```python
from build123d import *

# Parameters (mm, degrees)
BOSS_EXTRUDE1_DEPTH = 65
CUT_EXTRUDE1_DEPTH  = 40
CUT_EXTRUDE4_DEPTH  = 22.5
SKETCH6_R           = 12.5
SKETCH6_R_2         = 5
BOSS_EXTRUDE2_DEPTH = 12
CHAMFER1_SIZE       = 5
FILLET1_R           = 1
SKETCH7_R           = 1
CUT_EXTRUDE5_DEPTH  = 66


with BuildPart() as part:
    # Sketch1 → Boss-Extrude1 (new body, symmetric)
    with BuildSketch(Plane.XY):
        with BuildLine():
            Line((0, 0), (0, -25.554938316))
            ThreePointArc((0, -25.554938316), (-2.359933303, -32.007021768), (-8.325876175, -35.413807897))
            Line((-8.325876175, -35.413807897), (-67.775097409, -45.508814922))
            ThreePointArc((-67.775097409, -45.508814922), (-71.838201048, -44.399413479), (-73.612159322, -40.579380131))
            Line((-73.612159322, -40.579380131), (-73.612159322, -6.5))
            Line((-73.612159322, -6.5), (-29.367881905, -6.5))
            ThreePointArc((-29.367881905, -6.5), (-23.632117541, -4.691520443), (-19.970955697, 0.079798567))
            Line((-19.970955697, 0.079798567), (-20, 0))
            Line((-20, 0), (0, 0))
        make_face()
    extrude(amount=BOSS_EXTRUDE1_DEPTH, both=True)

    # Sketch2 → Cut-Extrude1 (cut, symmetric)
    with BuildSketch(Plane.XY):
        with BuildLine():
            Line((-20, 0), (-19.970955697, 0.079798567))
            ThreePointArc((-19.970955697, 0.079798567), (-20.672372291, -1.438432196), (-21.617003148, -2.818534521))
            Line((-21.617003148, -2.818534521), (-12.102051753, -36.055036129))
            Line((-12.102051753, -36.055036129), (-8.325876175, -35.413807897))
            ThreePointArc((-8.325876175, -35.413807897), (-2.359933303, -32.007021768), (0, -25.554938316))
            Line((0, -25.554938316), (0, 0))
            Line((0, 0), (-20, 0))
        make_face()
    extrude(amount=CUT_EXTRUDE1_DEPTH, both=True, mode=Mode.SUBTRACT)

    # Sketch5 → Cut-Extrude4 (cut, symmetric)
    with BuildSketch(Plane(origin=(0, -6.5, 0), x_dir=(1, 0, 0), z_dir=(0, 1, 0))):
        Polygon((-73.612159322, 40), (-29.401702386, 40), (0, 40), (0, -40), (-29.367881905, -40), (-73.612159322, -40), align=None)
    extrude(amount=CUT_EXTRUDE4_DEPTH, both=True, mode=Mode.SUBTRACT)

    # Sketch6 → Boss-Extrude2 (add)
    with BuildSketch(Plane(origin=(5.611689276, -33.047085202, 0), x_dir=(0.985886958, 0.167412383, 0), z_dir=(0.167412383, -0.985886958, 0))):
        with Locations((-42.967314491, 0)):
            Circle(SKETCH6_R)
        with Locations((-42.967314491, 0)):
            Circle(SKETCH6_R_2, mode=Mode.SUBTRACT)
    extrude(amount=BOSS_EXTRUDE2_DEPTH)

    # Chamfer1
    chamfer1_edges = [part.edges().sort_by_distance(p)[0] for p in [
        (-49.072812682, -42.333000474, 0),
    ]]
    chamfer(chamfer1_edges, length=CHAMFER1_SIZE)

    # Fillet1
    fillet1_edges = [part.edges().sort_by_distance(p)[0] for p in [
        (-54.002247473, -43.170062387, 0),
        (-47.063864092, -54.163643971, 0),
        (-48.23575077, -47.262435265, 0),
    ]]
    fillet(fillet1_edges, radius=FILLET1_R)

    # Sketch7 → Cut-Extrude5 (cut, through all)
    with BuildSketch(Plane.XY):
        with Locations((-34.907689498, -48.549314554)):
            Circle(SKETCH7_R)
    extrude(amount=-CUT_EXTRUDE5_DEPTH, mode=Mode.SUBTRACT)


solid = part.part
```
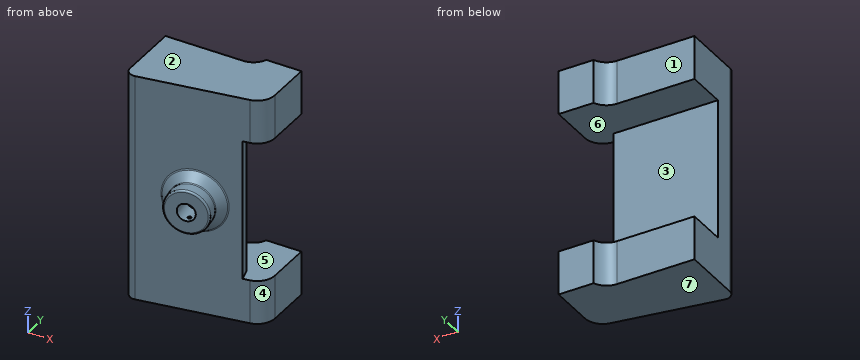
Here's how the part is built. I have some questions about the finished solid (model axes, mm). Face numbers are marked on the shaded views. A direction names the side the tool comes from. Give positions to 0.01 mm unless a question says otherwise; leave off trailing zeros. Write each loop counter-clockwise with the first axis right and the second up, starting at its lowest first coordinate (ties: lowest second). Pieces come first, ordered by that corner, then holes.
(1) On a 3-axis mill with a long thin cutter (end or side, diameter ignored), from which of +Z, -Z, +X, -X, +Y, -Y can I reach the whole of each face in a straight line? I mean the marked faces 1, 2 and 3. Say none if no direction works.
Output values:
face 1: +Z, -Z, -X, +Y
face 2: +Z, +X, -X, +Y, -Y
face 3: +X, -X, +Y
(2) Will these pins go through, and if not, where does the flat tip stop? pin 1 (10 mm diameter, centred on x = -10.5, z = 54.5, fed in from +Y); pin 2 (5 mm diameter, centred on x = -25.5, z = -28, fed in from +Y); pin 3 (7.5 mm diameter, centred on x = -47.5, z = 47, fed in from +Y); pin 4 (8 mm diameter, centred on y = -22.5, z = 39.5, fed in from -X).
Output values:
pin 1: stops at y = 0
pin 2: stops at y = -29
pin 3: stops at y = -6.5
pin 4: stops at x = -73.61
(3) Imagine slicing it at C-C, the plane y = -33. Write out the boundary of the cut face in (x, z).
Output values:
outline: (-73.61, -65) - (-3.32, -65) - (-3.32, -40) - (-12.98, -40) - (-12.98, 40) - (-3.32, 40) - (-3.32, 65) - (-73.61, 65) - close
(4) Imagine slicing it at D-D, the plane z = -28.5. Write out the boundary of the cut face in (x, y).
Output values:
outline: (-73.61, -40.58) arc R5 ccw to (-67.78, -45.51) - (-12.1, -36.06) - (-14.12, -29) - (-73.61, -29) - close
(5) If I drill on L1, parallel to Z at x = -20, y = -22.5; L2, parallel to Y at x = -69.5, z = 18.5; L3, parallel to Y at x = -23.5, z = 17, over which ranges is the centre line in solid material (lowest first)?
Output values:
L1: z = -65 to -40, 40 to 65
L2: y = -45.5 to -29
L3: y = -37.99 to -29
(6) Imagine slicing it at A-A, the plane y = -16.5. Write out the boundary of the cut face in (x, z).
Output values:
outline: (-73.61, -65) - (0, -65) - (0, -40) - (-73.61, -40) - close; (-73.61, 40) - (0, 40) - (0, 65) - (-73.61, 65) - close
(7) Thinking about a two-plate mould opening in Z: for the marked faces 4, 5, 6 and 7, which applies, pulls with the +Z half, pulls with the -Z half, needs draft (parallel to the pull), parting line crosses it, or undercut?
Output values:
face 4: needs draft
face 5: undercut
face 6: undercut
face 7: pulls with the -Z half
(8) Imagine slicing it at B-B, the plane z = -50. Write out the boundary of the cut face in (x, y).
Output values:
outline: (-73.61, -40.58) arc R5 ccw to (-67.78, -45.51) - (-8.33, -35.41) arc R10 ccw to (0, -25.55) - (0, 0) - (-20, 0) - (-19.97, 0.08) arc R10 cw to (-29.37, -6.5) - (-73.61, -6.5) - close
